The listing builds one solid part. Answer for the finished solid, in the listing's coordinates (mm). A direction names the side the tool comes from. Coordinates: 2 decimals unless noted, no trailing zeros. Write each loop counter-clockwise with the first axis right and the second up, starting at its lowest first coordinate (ties: lowest second). Pieces come first, ordered by that corner, then holes.
from build123d import *

# Parameters (mm, degrees)
F1_DEPTH = 78
F2_R     = 12
F4_D     = 8.5


with BuildPart() as f1:
    # F0 (on Front) → F1 (new body)
    with BuildSketch(Plane.XZ):
        Polygon((-33, 4), (-33, 0), (33, 0), (33, 4), (68, 4), (68, 16), (24, 16), (24, 12), (-24, 12), (-24, 16), (-68, 16), (-68, 4), align=None)
    extrude(amount=F1_DEPTH)

    # F2
    f2_edges = [f1.edges().sort_by_distance(p)[0] for p in [
        (-68, -78, 10),
        (68, -78, 10),
        (68, 0, 10),
        (-68, 0, 10),
    ]]
    fillet(f2_edges, radius=F2_R)

    # F4 (through all)
    with Locations(Plane.XY.offset(16)):
        with Locations((-56, -66), (-56, -12), (56, -66), (56, -12)):
            Hole(F4_D / 2)


solid = f1.part
Q1. Determine the mould class of faces 1 (the face through (52.074, -13.628, 9.916)), 2 (the face through (50, -38, 4)), 3 (the face through (-64.58, -74.39, 9.92)), 4 (the face through (-59.926, -13.628, 9.916)) for opening direction Y: released by +Y, released by -Y, zero draft, split by the parting line, or undercut.
Answers below:
face 1: undercut
face 2: zero draft
face 3: released by -Y
face 4: undercut
Q2. The part is cut by section A-A, the plane z = 14. Write down the section's boundary in (x, y).
Answers below:
outline: (-68, -66) arc R12 ccw to (-56, -78) - (-24, -78) - (-24, 0) - (-56, 0) arc R12 ccw to (-68, -12) - close; (24, -78) - (56, -78) arc R12 ccw to (68, -66) - (68, -12) arc R12 ccw to (56, 0) - (24, 0) - close; hole circle Ø8.5 at (-56, -66); hole circle Ø8.5 at (-56, -12); hole circle Ø8.5 at (56, -66); hole circle Ø8.5 at (56, -12)
Q3. The part is cut by section D-D, the plane z = 2.25. Write down the section's boundary in (x, y).
Answers below:
outline: (-33, -78) - (33, -78) - (33, 0) - (-33, 0) - close
Q4. The part is cut by section B-B, the plane y = -19.5. Write down the section's boundary in (x, z).
Answers below:
outline: (-68, 4) - (-33, 4) - (-33, 0) - (33, 0) - (33, 4) - (68, 4) - (68, 16) - (24, 16) - (24, 12) - (-24, 12) - (-24, 16) - (-68, 16) - close
Q5. Which of the six approach directions +Z, -Z, +X, -X, +Y, -Y give full straight-line access (tool end or side, diameter ignored) to faces 5 (the face through (-24, -38, 14)), 6 (the face through (-64.58, -3.61, 9.92)), 7 (the face through (-33, -38, 2))?
Answers below:
face 5: +Z, +Y, -Y
face 6: +Z, -Z, -X, +Y
face 7: -Z, -X, +Y, -Y
Q6. Given pin 1 (5 mm diameter, centred on x = -56, y = -12, fed in from -Z); pin 2 (4 mm diameter, centred on x = 13, y = -60.5, fed in from +Z); pin 3 (3 mm diameter, centred on y = -19.5, z = 1, fed in from +X); pin 4 (13.5 mm diameter, centred on x = 56, y = -12, fed in from +Z), each flat-ended and moving along its own axis, determine where each tip first touches the part or whether it passes through.
Answers below:
pin 1: passes through
pin 2: stops at z = 12
pin 3: stops at x = 33
pin 4: stops at z = 16
Q7. Find the intervals of material crossed by probe 1 along Y at (x, z) = (56, 11); probe 2 along X at (y, z) = (-14, 8); probe 3 along Z at (x, y) = (-41.5, -25), in increasing order.
Answers below:
probe 1: y = -78 to -70.25, -61.75 to -16.25, -7.75 to 0
probe 2: x = -68 to -59.75, -52.25 to 52.25, 59.75 to 68
probe 3: z = 4 to 16
Q8. The part is cut by section C-C, the plane x = 0. Write down the section's boundary in (y, z).
Answers below:
outline: (-78, 0) - (0, 0) - (0, 12) - (-78, 12) - close
